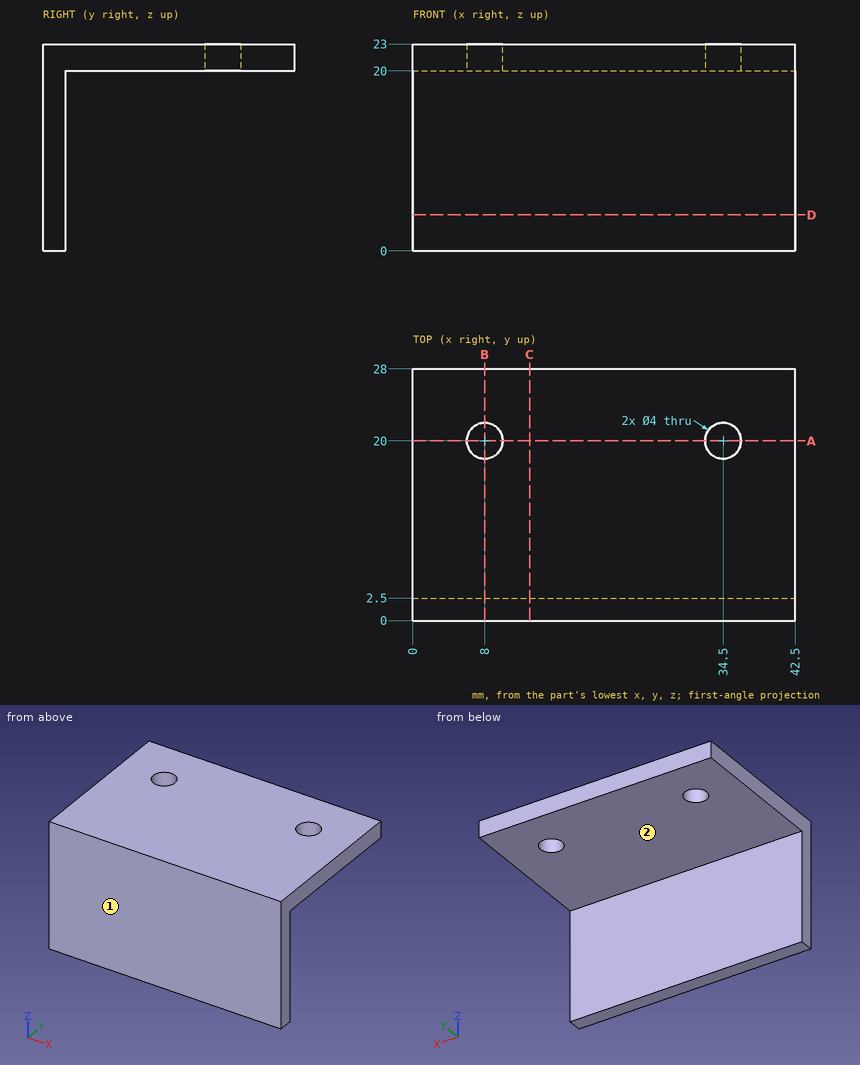
Here's the drawing with two shaded views (mm, measured from the low corner). I have some questions. A direction names the side the tool comes from. Coordinates: 2 decimals unless noted, no trailing zeros. Write each loop counter-clockwise with the first axis right and the second up, starting at its lowest first coordinate (ties: lowest second). Pieces come first, ordered by that corner, then holes.
Item 1: If I drill on line 1 (X direction, y = 20, z = 21.55); line 2 (Y direction, x = 34.5, z = 21.3); line 3 (Y direction, x = 3.5, z = 11.5), over which ranges is the centre line in solid material (lowest first)?
Item 2: Will these pins go through, and if not, where does the flat tip stop? pin 1 (7.5 mm diameter, centred on x = 15, y = 16.5, fed in from -Z); pin 2 (1.5 mm diameter, centred on x = 23, z = 14.5, fed in from +Y); pin 3 (3 mm diameter, centred on x = 8, y = 20, fed in from -Z).
Item 3: I want a section at D-D on z = 4. Write out the boundary of the cut face in (x, y).
Item 4: I want a section at C-C on x = 13. Write out the boundary of the cut face in (y, z), and give its area (3 significant figures).
Item 5: I want a section at B-B on x = 8. Write out the boundary of the cut face in (y, z).
Item 6: On a 3-axis mill with a long thin cutter (end or side, diameter ignored), from which of +Z, -Z, +X, -X, +Y, -Y can I reach the whole of each face in a straight line? I mean the marked faces 1 and 2. Say none if no direction works.
Item 7: I want a section at A-A on y = 20. Write out the boundary of the cut face in (x, z).
Findings below:
1. line 1: x = 0 to 6, 10 to 32.5, 36.5 to 42.5
1. line 2: y = 0 to 18, 22 to 28
1. line 3: y = 0 to 2.5
2. pin 1: stops at z = 20
2. pin 2: stops at y = 2.5
2. pin 3: passes through
3. outline: (0, 0) - (42.5, 0) - (42.5, 2.5) - (0, 2.5) - close
4. outline: (0, 0) - (2.5, 0) - (2.5, 20) - (28, 20) - (28, 23) - (0, 23) - close
4. area: 134 mm2
5. outline: (0, 0) - (2.5, 0) - (2.5, 20) - (18, 20) - (18, 23) - (0, 23) - close; (22, 20) - (28, 20) - (28, 23) - (22, 23) - close
6. face 1: +Z, -Z, +X, -X, -Y
6. face 2: -Z, +X, -X, +Y
7. outline: (0, 20) - (6, 20) - (6, 23) - (0, 23) - close; (10, 20) - (32.5, 20) - (32.5, 23) - (10, 23) - close; (36.5, 20) - (42.5, 20) - (42.5, 23) - (36.5, 23) - close
